Drawing for the job (mm, zero at the part's lowest x, y, z). A direction names the side the tool comes from. Give positions to 0.01 mm unless a question says otherwise; leave off trailing zeros. Write each loop counter-clockwise with the first axis right and the second up, starting at its lowest first coordinate (ties: lowest second). Pieces come first, ordered by that corner, then holes.
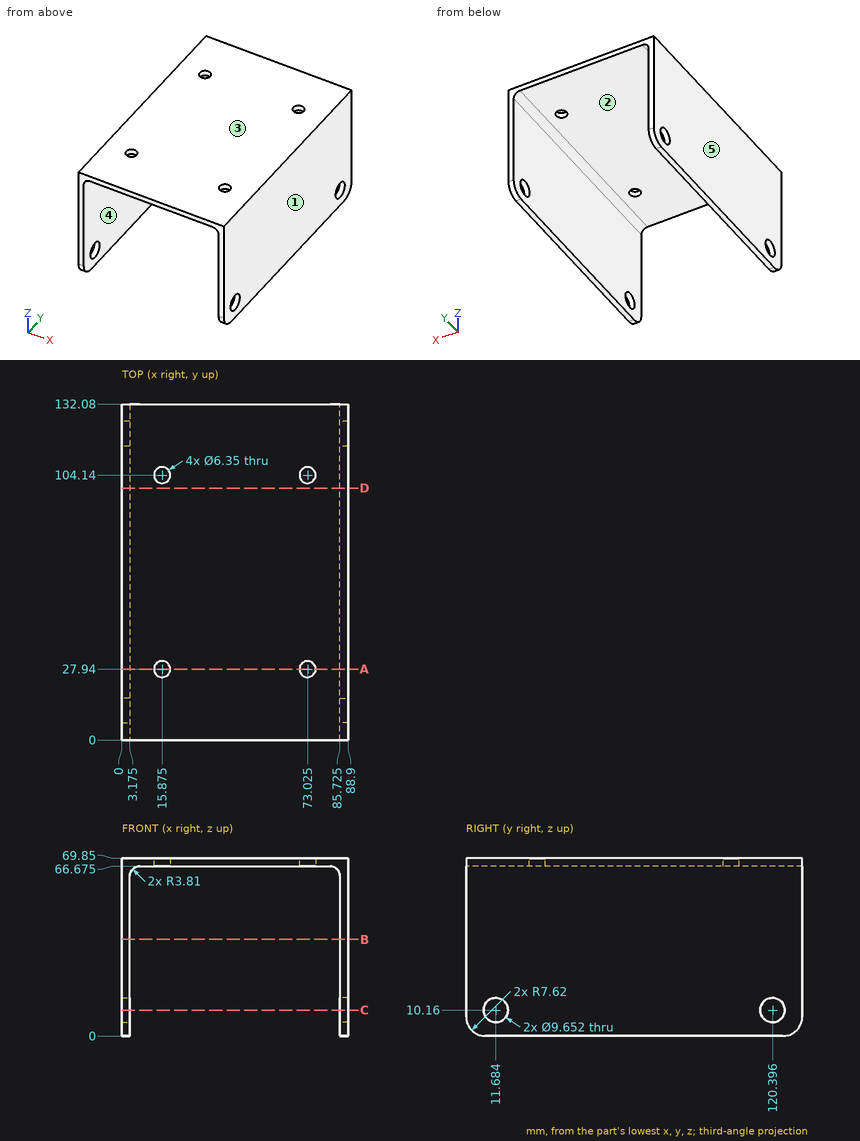
1. Which spindle directions (+Z, -Z, +X, -X, +Y, -Y) get a long thin tool onto all of the face, cutting with end or side? Do the marked faces 4 and 5. Say none if no direction does.
Calculated:
face 4: -Z, +Y, -Y
face 5: +Z, -Z, -X, +Y, -Y
2. Pin check, flat tip, straight feed: P1, Ø22.5, axis at x = 49.5, y = 79, coming from the -Z side (3 decimals). Stop position of the tip, or through.
Calculated:
P1: stops at z = 66.675
3. Slice it at B-B, the plane z = 38. Write the cut outline in (x, y) (3 decimals).
Calculated:
outline: (0, 0) - (3.175, 0) - (3.175, 132.08) - (0, 132.08) - close; (85.725, 0) - (88.9, 0) - (88.9, 132.08) - (85.725, 132.08) - close
4. Probe probe 1 along X at (y, z) = (104, 69); probe 2 along X at (y, z) = (75.5, 37) (3 decimals); probe 3 along Z at (x, y) = (71, 60.5) (3 decimals). List the from-to ranges inside material, lowest first.
Calculated:
probe 1: x = 0 to 12.7, 19.05 to 69.85, 76.2 to 88.9
probe 2: x = 0 to 3.175, 85.725 to 88.9
probe 3: z = 66.675 to 69.85
5. Pull direction X, two halves, no side cores. Call the marked faces 1, 2 and 3: +X half, -X half, draft (parallel to the pull), parting line (faces both ways), or undercut.
Calculated:
face 1: +X half
face 2: undercut
face 3: draft
6. Slice it at A-A, the plane y = 27.94. Write the cut outline in (x, z) (3 decimals).
Calculated:
outline: (0, 0) - (3.175, 0) - (3.175, 62.865) arc R3.81 cw to (6.985, 66.675) - (12.7, 66.675) - (12.7, 69.85) - (0, 69.85) - close; (19.05, 66.675) - (69.85, 66.675) - (69.85, 69.85) - (19.05, 69.85) - close; (76.2, 66.675) - (81.915, 66.675) arc R3.81 cw to (85.725, 62.865) - (85.725, 0) - (88.9, 0) - (88.9, 69.85) - (76.2, 69.85) - close
7. Slice it at C-C, the plane z = 10.16. Write the cut outline in (x, y) (3 decimals).
Calculated:
outline: (0, 0) - (3.175, 0) - (3.175, 6.858) - (0, 6.858) - close; (0, 16.51) - (3.175, 16.51) - (3.175, 115.57) - (0, 115.57) - close; (0, 125.222) - (3.175, 125.222) - (3.175, 132.08) - (0, 132.08) - close; (85.725, 0) - (88.9, 0) - (88.9, 6.858) - (85.725, 6.858) - close; (85.725, 16.51) - (88.9, 16.51) - (88.9, 115.57) - (85.725, 115.57) - close; (85.725, 125.222) - (88.9, 125.222) - (88.9, 132.08) - (85.725, 132.08) - close
8. Slice it at D-D, the plane y = 99. Write the cut outline in (x, z) (3 decimals), and give its area (3 significant figures).
Calculated:
outline: (0, 0) - (3.175, 0) - (3.175, 62.865) arc R3.81 cw to (6.985, 66.675) - (81.915, 66.675) arc R3.81 cw to (85.725, 62.865) - (85.725, 0) - (88.9, 0) - (88.9, 69.85) - (0, 69.85) - close
area: 712 mm2
